```python
from build123d import *

# Parameters (mm, degrees)
F0_W     = 25
F0_H     = 20
F1_DEPTH = 70
F3_DEPTH = 21
F4_W     = 50
F4_H     = 40
F5_DEPTH = 4
F6_R     = 1


with BuildPart() as f1:
    # F0 (on Top) → F1 (new body)
    with BuildSketch(Plane.XY):
        Rectangle(F0_W, F0_H)
    extrude(amount=F1_DEPTH)

    # F2 (on face) → F3 (cut)
    with BuildSketch(Plane.YZ.offset(12.5)):
        Polygon((7.25, 70), (-7.25, 70), (-7.25, 68.4), (-6.25, 68.4), (-6.25, 28.4), (6.25, 28.4), (6.25, 68.4), (7.25, 68.4), align=None)
    extrude(amount=-F3_DEPTH, mode=Mode.SUBTRACT)

    # F4 (on face) → F5 (join)
    with BuildSketch(Plane(origin=(0, 0, 0), x_dir=(1, 0, 0), z_dir=(0, 0, -1))):
        Rectangle(F4_W, F4_H)
    extrude(amount=-F5_DEPTH)

    # F6
    f6_edges = [f1.edges().sort_by_distance(p)[0] for p in [
        (0, 20, 4),
        (-25, 0, 4),
        (25, 0, 4),
        (0, -20, 4),
        (0, -10, 4),
        (-12.5, 0, 4),
        (0, 10, 4),
        (12.5, 0, 4),
        (12.5, 10, 37),
        (12.5, 8.625, 70),
        (12.5, 7.25, 69.2),
        (12.5, 6.75, 68.4),
        (12.5, 6.25, 48.4),
        (12.5, 0, 28.4),
        (12.5, -6.25, 48.4),
        (12.5, -6.75, 68.4),
        (12.5, -7.25, 69.2),
        (12.5, -8.625, 70),
        (12.5, -10, 37),
        (-12.5, 10, 37),
        (0, 10, 70),
        (-12.5, -10, 37),
        (-12.5, 0, 70),
        (0, -10, 70),
    ]]
    fillet(f6_edges, radius=F6_R)


solid = f1.part
```
The model under review builds one solid part; all positions refer to its coordinate system, in mm. A direction names the side the tool comes from. Round coordinates to 2 decimals unless told otherwise and drop trailing zeros. Loops run counter-clockwise (first coordinate to the right, second up) from the corner with the lowest first, then second, coordinate; pieces in that order, holes last. Notation, with made-up numbers: (-26.75, 87.25) - (-9.75, 87.25) arc R11 cw to (-9.75, 92.25) - close; hole circle Ø6 at (67, 7). An arc over 180 degrees is marked (long way). Use a Markdown table: item, result. Add a question column.
Q1. For probe 1 along Y at (x, z) = (-5.5, 35.5); probe 2 along Z at (x, y) = (-0.5, 15); probe 3 along X at (y, z) = (7.5, 5), list the stretches that pass through material, from the lowest coordinate up.
Q2. Insertion check: pin 1 Ø22 at (x, z) = (-0.5, 48.5) entering from -Y; pin 2 Ø2 at (y, z) = (-6, 60) entering from +X; pin 3 Ø9 at (y, z) = (0.5, 42) entering from -X; pin 4 Ø12 at (x, z) = (0.5, 8) entering from +Y. Each pin has a flat end and moves straight along its axis. Give the tip position at first contact, or say it passes through.
Q3. Add section B-B (z = 6). State the section outline as (x, y) points, plus the area to 3 significant figures.
Q4. Add section D-D (z = 30). State the section outline as (x, y) points, plus the area to 3 significant figures.
Q5. Add section C-C (y = -5). State the section outline as (x, z) points, plus the area to 3 significant figures.
Q6. Add section A-A (x = -3.5). State the section outline as (y, z) points, plus the area to 3 significant figures.
Q7. The part is to be moulded in two halves that separate along Y. For faces 4 (the face through (0, -10, 37)), 5 (the face through (2, -7.25, 69)), 6 (the face through (-9, -1, 70)), say which applies: pulls with the +Y half, pulls with the -Y half, needs draft (parallel to the pull), parting line crosses it, or undercut.
Q8. Machinability: for faces 1 (the face through (0, -13, 4)), 2 (the face through (2, 7.25, 69)), 3 (the face through (0, 10, 37)), which of the approach directions +Z, -Z, +X, -X, +Y, -Y give a long, thin tool a straight path to every point of the face, cutting with its end or side? Answer none if there is none.
Worked answers:
| question | item | result |
|---|---|---|
| 1 | probe 1 | -10 to -6.25, 6.25 to 10 |
| 1 | probe 2 | 0 to 4 |
| 1 | probe 3 | -12.5 to 12.5 |
| 2 | pin 1 | y = -10 |
| 2 | pin 2 | x = 12.47 |
| 2 | pin 3 | x = -12.5 |
| 2 | pin 4 | y = 20 |
| 3 | outline | (-12.5, -9) arc R1 ccw to (-11.5, -10) - (11.5, -10) arc R1 ccw to (12.5, -9) - (12.5, 9) arc R1 ccw to (11.5, 10) - (-11.5, 10) arc R1 ccw to (-12.5, 9) - close |
| 3 | area | 499 mm² |
| 4 | outline | (-12.5, -9) arc R1 ccw to (-11.5, -10) - (11.5, -10) arc R1 ccw to (12.5, -9) - (12.5, -7.25) arc R1 ccw to (11.5, -6.25) - (-8.5, -6.25) - (-8.5, 6.25) - (11.5, 6.25) arc R1 ccw to (12.5, 7.25) - (12.5, 9) arc R1 ccw to (11.5, 10) - (-11.5, 10) arc R1 ccw to (-12.5, 9) - close |
| 4 | area | 236 mm² |
| 5 | outline | (-25, 0) - (25, 0) - (25, 3) arc R1 ccw to (24, 4) - (13.5, 4) arc R1 cw to (12.5, 5) - (12.5, 27.4) arc R1 ccw to (11.5, 28.4) - (-8.5, 28.4) - (-8.5, 70) - (-11.5, 70) arc R1 ccw to (-12.5, 69) - (-12.5, 5) arc R1 cw to (-13.5, 4) - (-24, 4) arc R1 ccw to (-25, 3) - close |
| 5 | area | 976 mm² |
| 6 | outline | (-20, 0) - (20, 0) - (20, 3) arc R1 ccw to (19, 4) - (11, 4) arc R1 cw to (10, 5) - (10, 69) arc R1 ccw to (9, 70) - (7.25, 70) - (7.25, 68.4) - (6.25, 68.4) - (6.25, 28.4) - (-6.25, 28.4) - (-6.25, 68.4) - (-7.25, 68.4) - (-7.25, 70) - (-9, 70) arc R1 ccw to (-10, 69) - (-10, 5) arc R1 cw to (-11, 4) - (-19, 4) arc R1 ccw to (-20, 3) - close |
| 6 | area | 956 mm² |
| 7 | face 4 | pulls with the -Y half |
| 7 | face 5 | undercut |
| 7 | face 6 | needs draft |
| 8 | face 1 | +Z |
| 8 | face 2 | +Z, +X |
| 8 | face 3 | +Z, +X, -X, +Y |
